Read the model definition and answer for the solid it produces. Units are mm, in the model's axes. A direction names the side the tool comes from. Coordinates: 2 decimals unless noted, no trailing zeros. Order: outer loops, then holes, each group sorted by start corner. A loop starts at its lowest first (then second) coordinate and runs counter-clockwise, first axis right, second up. Notation, with made-up numbers: M -12.5,47.5 L 9.5,47.5 A30 cw 9.5,77.5 Z; hole C 67.5,73.25 d10. An arc over 180 degrees is marked long. Put each result on its own line as item: value.
from build123d import *

# Parameters (mm, degrees)
SKETCH1_R           = 34
BOSS_EXTRUDE1_DEPTH = 180
SKETCH2_R           = 27.5
CUT_EXTRUDE1_DEPTH  = 181
SKETCH3_R           = 28.5
SKETCH3_R_2         = 27.5
CUT_EXTRUDE2_DEPTH  = 2


with BuildPart() as part:
    # Sketch1 → Boss-Extrude1 (new body)
    with BuildSketch(Plane(origin=(0, 0, 0), x_dir=(1, 0, 0), z_dir=(0, 1, 0))):
        Circle(SKETCH1_R)
    extrude(amount=BOSS_EXTRUDE1_DEPTH)

    # Sketch2 → Cut-Extrude1 (cut, through all)
    with BuildSketch(Plane.XZ):
        Circle(SKETCH2_R)
    extrude(amount=-CUT_EXTRUDE1_DEPTH, mode=Mode.SUBTRACT)

    # Sketch3 → Cut-Extrude2 (cut)
    with BuildSketch(Plane(origin=(0, 39, 0), x_dir=(-1, 0, 0), z_dir=(0, -1, 0))):
        Circle(SKETCH3_R)
        Circle(SKETCH3_R_2, mode=Mode.SUBTRACT)
    extrude(amount=CUT_EXTRUDE2_DEPTH, mode=Mode.SUBTRACT)


solid = part.part
Q1. For a pull along Y with two mould halves and no side action, classify faces 3 (the face through (14.9, 37, -23.4)), 4 (the face through (28, 0, 0)), 5 (the face through (28, 180, 0)), 6 (the face through (-5.961, 18.241, -26.846)) as +Y half, -Y half, draft (parallel to the pull), parting line (faces both ways), or undercut.
Answers below:
face 3: undercut
face 4: -Y half
face 5: +Y half
face 6: draft
Q2. Find section C-C on y = 103. Write down the section's boundary in (x, z).
Answers below:
outline: C 0,0 d68; hole C 0,0 d55
Q3. Given pin 1 (4 mm diameter, centred on y = 136.5, z = 5, fed in from -X); pin 2 (1 mm diameter, centred on y = 21, z = -6.5, fed in from +X); pin 3 (5 mm diameter, centred on x = -23, y = 43, fed in from +Z); pin 4 (4 mm diameter, centred on x = 26, z = 19, fed in from -Y), each flat-ended and moving along its own axis, determine where each tip first touches the part or whether it passes through.
Answers below:
pin 1: stops at x = -33.87
pin 2: stops at x = 33.47
pin 3: stops at z = 27.12
pin 4: stops at y = 0
Q4. Find section B-B on x = 0. Write down the section's boundary in (y, z), plus the area to 3 significant figures.
Answers below:
outline: M 0,-34 L 180,-34 L 180,-27.5 L 39,-27.5 L 39,-28.5 L 37,-28.5 L 37,-27.5 L 0,-27.5 Z; M 0,27.5 L 37,27.5 L 37,28.5 L 39,28.5 L 39,27.5 L 180,27.5 L 180,34 L 0,34 Z
area: 2,340 mm^2
Q5. A tool of negligible diameter and unlimited length cuts with its end or side. For faces 1 (the face through (14.9, 39, -23.4)), 2 (the face through (18.28, 88.74, -28.67)), from which of +Z, -Z, +X, -X, +Y, -Y can it reach the whole face along a straight path? Write none if from no direction.
Answers below:
face 1: none
face 2: +Y, -Y
Q6. Find section A-A on z = 0. Write down the section's boundary in (x, y), plus the area to 3 significant figures.
Answers below:
outline: M -34,0 L -27.5,0 L -27.5,37 L -28.5,37 L -28.5,39 L -27.5,39 L -27.5,180 L -34,180 Z; M 27.5,0 L 34,0 L 34,180 L 27.5,180 L 27.5,39 L 28.5,39 L 28.5,37 L 27.5,37 Z
area: 2,340 mm^2
Q7. Consider line 1 along X through (y, z) = (172.5, 1); line 2 along Z through (x, y) = (0, 21); line 3 along X through (y, z) = (90, -18). Determine where each line is inside the solid, lowest interval first.
Answers below:
line 1: x = -33.99 to -27.48, 27.48 to 33.99
line 2: z = -34 to -27.5, 27.5 to 34
line 3: x = -28.84 to -20.79, 20.79 to 28.84
